Job drawing, mm, ordinate dimensions from the low corner. One solid piece. Give positions to 0.01 mm unless a question says otherwise; leave off trailing zeros. Order: outer loops, then holes, each group sorted by start corner. A loop starts at its lowest first (then second) coordinate and runs counter-clockwise, first axis right, second up. Notation, with made-up numbers: M 71.5,86.5 L 112.5,86.5 A18 ccw 112.5,94.5 Z; hole C 84.25,49 d7. An arc over 180 degrees is marked long. One line per question, with ' | ' between items.
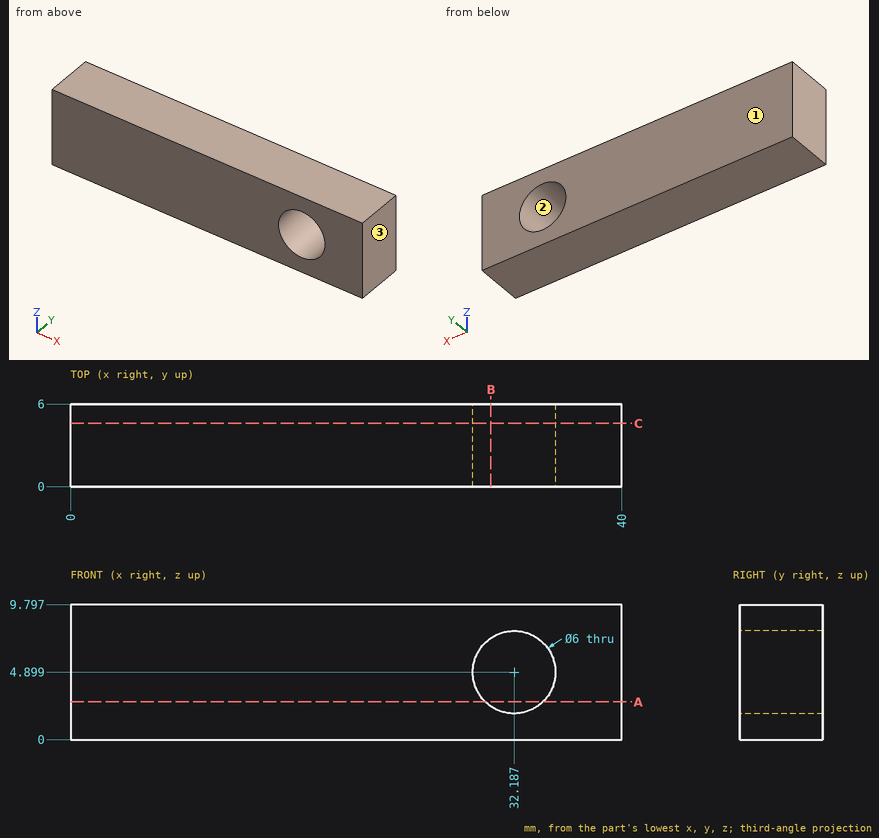
1. Probe L1, parallel to X at y = 5.7, z = 7 (1 decimal); L2, parallel to Z at x = 33.5, y = 2.2 (1 decimal); L3, parallel to X at y = 1.85, z = 4.5. List the from-to ranges inside material, lowest first. Write a range as from..to.
Worked out:
L1: x = 0..30, 34.3..40 | L2: z = 0..2.2, 7.6..9.8 | L3: x = 0..29.21, 35.16..40
2. Slice it at A-A on z = 2.75. Give the cut face in (x, y).
Worked out:
outline: M 0,0 L 30.09,0 L 30.09,6 L 0,6 Z; M 34.28,0 L 40,0 L 40,6 L 34.28,6 Z
3. Slice it at C-C on y = 4.6. Give the cut face in (x, z).
Worked out:
outline: M 0,0 L 40,0 L 40,9.8 L 0,9.8 Z; hole C 32.19,4.9 d6
4. Slice it at B-B on x = 30.5. Give the cut face in (y, z), then the cut area to 3 significant figures.
Worked out:
outline: M 0,0 L 6,0 L 6,2.42 L 0,2.42 Z; M 0,7.38 L 6,7.38 L 6,9.8 L 0,9.8 Z | area: 29.0 mm2
5. Mould opens along X. For the marked faces 1, 2 and 3 say: released by +X, released by -X, zero draft, split by the parting line, or undercut.
Worked out:
face 1: zero draft | face 2: undercut | face 3: released by +X
